The listing builds one solid part. Answer for the finished solid, in the listing's coordinates (mm). Give positions to 0.01 mm unless a question says otherwise; leave off trailing zeros. Loops run counter-clockwise (first coordinate to the right, second up) from the corner with the lowest first, then second, coordinate; pieces in that order, holes last. Notation, with made-up numbers: (46.5, 5.25) - (87.5, 5.25) arc R13 ccw to (87.5, 25.25) - close; hole circle Ø4 at (-26, 35.25). An arc over 180 degrees is marked (long way). Answer in a Markdown table with one row per item. Add a question column.
```python
from build123d import *

# Parameters (mm, degrees)
SKETCH1_R           = 2
SKETCH1_R_2         = 2.1
SKETCH1_W           = 352.775
SKETCH1_H           = 95.6
BOSS_EXTRUDE1_DEPTH = 3


with BuildPart() as part:
    # Sketch1 → Boss-Extrude1 (new body)
    with BuildSketch(Plane(origin=(0, 0, 0), x_dir=(1, 0, 0), z_dir=(0, 1, 0))):
        with BuildLine():
            Line((4.973e-06, 108.600001742), (4.973e-06, 5.000001742))
            ThreePointArc((4.973e-06, 5.000001742), (1.464471067, 1.464467836), (5.000004973, 1.742e-06))
            Line((5.000004973, 1.742e-06), (365.775004973, 1.742e-06))
            ThreePointArc((365.775004973, 1.742e-06), (369.310538879, 1.464467836), (370.775004973, 5.000001742))
            Line((370.775004973, 5.000001742), (370.775004973, 108.600001742))
            ThreePointArc((370.775004973, 108.600001742), (369.310538879, 112.135535647), (365.775004973, 113.600001742))
            Line((365.775004973, 113.600001742), (5.000004973, 113.600001742))
            ThreePointArc((5.000004973, 113.600001742), (1.464471067, 112.135535647), (4.973e-06, 108.600001742))
        make_face()
        with Locations(Location((85.387504973, 107.600001742, 0), (0, 0, 270))):
            Circle(SKETCH1_R, mode=Mode.SUBTRACT)
        with Locations(Location((285.387504973, 107.600001742, 0), (0, 0, 270))):
            Circle(SKETCH1_R, mode=Mode.SUBTRACT)
        with Locations(Location((85.387504973, 6.000001741, 0), (0, 0, 270))):
            Circle(SKETCH1_R, mode=Mode.SUBTRACT)
        with Locations(Location((185.387504973, 6.000001741, 0), (0, 0, 270))):
            Circle(SKETCH1_R, mode=Mode.SUBTRACT)
        with Locations(Location((285.387504973, 6.000001741, 0), (0, 0, 270))):
            Circle(SKETCH1_R, mode=Mode.SUBTRACT)
        with Locations(Location((175.387504973, 109.100001742, 0), (0, 0, 270))):
            Circle(SKETCH1_R_2, mode=Mode.SUBTRACT)
        with Locations(Location((195.387504973, 109.100001742, 0), (0, 0, 270))):
            Circle(SKETCH1_R_2, mode=Mode.SUBTRACT)
        with Locations((185.387504973, 56.800001742)):
            Rectangle(SKETCH1_W, SKETCH1_H, mode=Mode.SUBTRACT)
        Polygon((234.088466868, 111.350001742), (236.686543079, 111.350001742), (237.985581185, 109.100001742), (236.686543079, 106.850001742), (234.088466868, 106.850001742), (232.789428762, 109.100001742), align=None, mode=Mode.SUBTRACT)
        Polygon((334.088466868, 111.350001742), (336.686543079, 111.350001742), (337.985581185, 109.100001742), (336.686543079, 106.850001742), (334.088466868, 106.850001742), (332.789428762, 109.100001742), align=None, mode=Mode.SUBTRACT)
        Polygon((365.947436577, 110.609550653), (367.784553885, 108.772433346), (367.11212228, 106.262884434), (364.602573369, 105.59045283), (362.765456062, 107.427570137), (363.437887666, 109.937119049), align=None, mode=Mode.SUBTRACT)
        Polygon((136.686543079, 111.350001742), (134.088466868, 111.350001742), (132.789428762, 109.100001742), (134.088466868, 106.850001742), (136.686543079, 106.850001742), (137.985581185, 109.100001742), align=None, mode=Mode.SUBTRACT)
        Polygon((36.686543079, 111.350001742), (34.088466868, 111.350001742), (32.789428762, 109.100001742), (34.088466868, 106.850001742), (36.686543079, 106.850001742), (37.985581185, 109.100001742), align=None, mode=Mode.SUBTRACT)
        Polygon((4.827573369, 110.609550653), (2.990456062, 108.772433346), (3.662887666, 106.262884434), (6.172436577, 105.59045283), (8.009553885, 107.427570137), (7.33712228, 109.937119049), align=None, mode=Mode.SUBTRACT)
        Polygon((234.088466868, 2.250001742), (236.686543079, 2.250001742), (237.985581185, 4.500001742), (236.686543079, 6.750001742), (234.088466868, 6.750001742), (232.789428762, 4.500001742), align=None, mode=Mode.SUBTRACT)
        Polygon((334.088466868, 2.250001742), (336.686543079, 2.250001742), (337.985581185, 4.500001742), (336.686543079, 6.750001742), (334.088466868, 6.750001742), (332.789428762, 4.500001742), align=None, mode=Mode.SUBTRACT)
        Polygon((365.947436577, 2.99045283), (367.784553885, 4.827570137), (367.11212228, 7.337119049), (364.602573369, 8.009550653), (362.765456062, 6.172433346), (363.437887666, 3.662884434), align=None, mode=Mode.SUBTRACT)
        Polygon((136.686543079, 2.250001742), (134.088466868, 2.250001742), (132.789428762, 4.500001742), (134.088466868, 6.750001742), (136.686543079, 6.750001742), (137.985581185, 4.500001742), align=None, mode=Mode.SUBTRACT)
        Polygon((36.686543079, 2.250001742), (34.088466868, 2.250001742), (32.789428762, 4.500001742), (34.088466868, 6.750001742), (36.686543079, 6.750001742), (37.985581185, 4.500001742), align=None, mode=Mode.SUBTRACT)
        Polygon((4.827573369, 2.99045283), (2.990456062, 4.827570137), (3.662887666, 7.337119049), (6.172436577, 8.009550653), (8.009553885, 6.172433346), (7.33712228, 3.662884434), align=None, mode=Mode.SUBTRACT)
    extrude(amount=-BOSS_EXTRUDE1_DEPTH)


solid = part.part
```
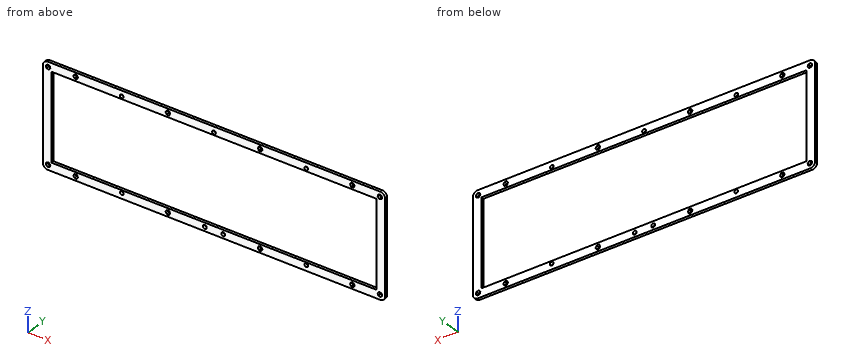
(1) Find the intervals of material crossed by line 1 along Z through (x, y) = (195.5, -0.25); line 2 along Z through (x, y) = (218, -0.95); line 3 along Z through (x, y) = (35, -0.35), in increasing order. Write a range as [from, to].
(2) A cutting plane is placed at A-A on z = -66.5. Determine the outline of the cut face in (x, y) (3 decimals), plus the area to 3 significant figures.
(3) A cutting plane is placed at B-B on x = 211. Determine the outline of the cut face in (y, z).
(4) A cutting plane is placed at C-C on y = -1.4. Give the number of separate pieces and of enclosed holes in the cut face, plus the area to 3 significant figures.
(5) Given pin 1 Ø2.5 at (x, z) = (195.39, -109.1) entering from +Y, flat-ended and moving along its own axis, determine where the tip first touches the part or whether it passes through.
Evaluation:
| question | item | result |
|---|---|---|
| 1 | line 1 | z = [-113.6, -111.2], [-107, -104.6], [-9, 0] |
| 1 | line 2 | z = [-113.6, -104.6], [-9, 0] |
| 1 | line 3 | z = [-113.6, -111.35], [-106.85, -104.6], [-9, -6.75], [-2.25, 0] |
| 2 | outline | (0, -3) - (9, -3) - (9, 0) - (0, 0) - close; (361.775, -3) - (370.775, -3) - (370.775, 0) - (361.775, 0) - close |
| 2 | area | 54.0 mm² |
| 3 | outline | (-3, -113.6) - (0, -113.6) - (0, -104.6) - (-3, -104.6) - close; (-3, -9) - (0, -9) - (0, 0) - (-3, 0) - close |
| 4 | separate pieces | 1 |
| 4 | enclosed holes | 20 |
| 4 | area | 8,070 mm² |
| 5 | pin 1 | passes through |
